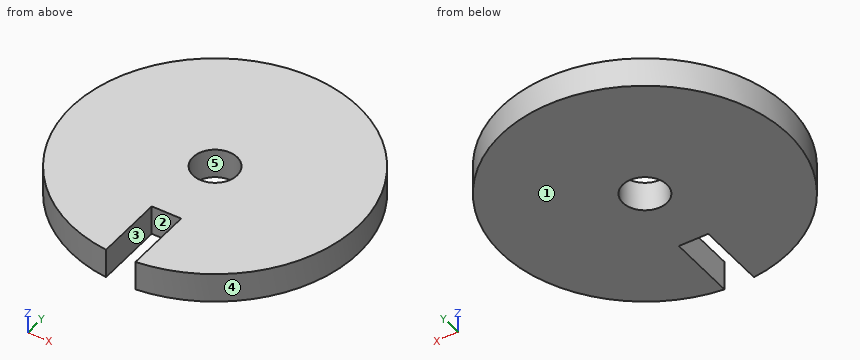
from build123d import *

# Parameters (mm, degrees)
SKIZZE1_R                       = 19.5
AUFSATZ_LINEAR_AUSTRAGEN1_DEPTH = 4
SKIZZE4_R                       = 3
SCHNITT_LINEAR_AUSTRAGEN2_DEPTH = 4
SKIZZE6_W                       = 4
SKIZZE6_H                       = 10
SCHNITT_LINEAR_AUSTRAGEN3_DEPTH = 4


with BuildPart() as part:
    # Skizze1 → Aufsatz-Linear austragen1 (new body)
    with BuildSketch(Plane.XY):
        Circle(SKIZZE1_R)
    extrude(amount=AUFSATZ_LINEAR_AUSTRAGEN1_DEPTH)

    # Skizze4 → Schnitt-Linear austragen2 (cut)
    with BuildSketch(Plane.XY.offset(4)):
        Circle(SKIZZE4_R)
    extrude(amount=-SCHNITT_LINEAR_AUSTRAGEN2_DEPTH, mode=Mode.SUBTRACT)

    # Skizze6 → Schnitt-Linear austragen3 (cut)
    with BuildSketch(Plane.XY.offset(4)):
        with Locations((0, -15)):
            Rectangle(SKIZZE6_W, SKIZZE6_H)
    extrude(amount=-SCHNITT_LINEAR_AUSTRAGEN3_DEPTH, mode=Mode.SUBTRACT)


solid = part.part
Build history of the part. All positions in model axes, mm. Face numbers are marked on the shaded views. A direction names the side the tool comes from. Round coordinates to 2 decimals unless told otherwise and drop trailing zeros. Write each loop counter-clockwise with the first axis right and the second up, starting at its lowest first coordinate (ties: lowest second). Pieces come first, ordered by that corner, then holes. Notation, with made-up numbers: M 56,59.5 L 68,59.5 A25 ccw 68,71.5 Z; hole C -23,10.25 d2. An arc over 180 degrees is marked long. Answer as a JSON object with one key per item and string values. Group by question number.
(1) Mould opens along Y. For the marked faces 3, 4 and 5 say: pulls with the +Y half, pulls with the -Y half, needs draft (parallel to the pull), parting line crosses it, or undercut.
(2) Which spindle directions (+Z, -Z, +X, -X, +Y, -Y) get a long thin tool onto all of the face, cutting with end or side? Do the marked faces 1 and 2. Say none if no direction does.
(3) Drill centre lines: L1, parallel to Y at x = 0, z = 3.2; L2, parallel to X at y = -14, z = 2.4; L3, parallel to X at y = -13.5, z = 3.4. Where is each one in solid material? Low to high.
(4) Cut at A-A (y = 0). Give the cut face in (x, z).
(5) Cut at C-C (x = 0). Give the cut face in (y, z).
(6) Flat gauge pins, fed straight in: pin 1 (1.5 mm diameter, centred on x = -12.5, z = 1.5, fed in from +Y); pin 2 (2 mm diameter, centred on x = 9, z = 3, fed in from -Y); pin 3 (2 mm diameter, centred on y = 15, z = 3, fed in from +X). Where does each tip first touch, or does it go through?
(7) Cut at D-D (x = 8). Give the cut face in (y, z), and give its area (3 significant figures).
(8) Cut at B-B (z = 0.8). Give the cut face in (x, y).
Responses:
{
 "1": {"face 3": "needs draft", "face 4": "parting line crosses it", "face 5": "undercut"},
 "2": {"face 1": "-Z, +X, -X, +Y, -Y", "face 2": "+Z, -Z, -Y"},
 "3": {"L1": "y = -10 to -3, 3 to 19.5", "L2": "x = -13.57 to -2, 2 to 13.57", "L3": "x = -14.07 to -2, 2 to 14.07"},
 "4": {"outline": "M -19.5,0 L -3,0 L -3,4 L -19.5,4 Z; M 3,0 L 19.5,0 L 19.5,4 L 3,4 Z"},
 "5": {"outline": "M -10,0 L -3,0 L -3,4 L -10,4 Z; M 3,0 L 19.5,0 L 19.5,4 L 3,4 Z"},
 "6": {"pin 1": "stops at y = 15.56", "pin 2": "stops at y = -17.78", "pin 3": "stops at x = 13.57"},
 "7": {"outline": "M -17.78,0 L 17.78,0 L 17.78,4 L -17.78,4 Z", "area": "142 mm2"},
 "8": {"outline": "M -2,-19.4 L -2,-10 L 2,-10 L 2,-19.4 A19.5 ccw long Z; hole C 0,0 d6"}
}
